from build123d import *
from build123d.topology import SkipClean

# Parameters (mm, degrees)
SKETCH2_W            = 55
SKETCH2_H            = 59
SKETCH2_R            = 1.6
SKETCH2_R_2          = 11
BOSS_EXTRUDE1_DEPTH  = 5
SKETCH4_W            = 5
SKETCH4_H            = 59
BOSS_EXTRUDE2_DEPTH  = 50
BOSS_EXTRUDE3_DEPTH  = 4
FILLET2_R            = 5
SKETCH7_W            = 5
SKETCH7_H            = 50
BOSS_EXTRUDE4_DEPTH  = 5
BOSS_EXTRUDE5_START  = -60
SKETCH8_W            = 5
SKETCH8_H            = 5
BOSS_EXTRUDE5_DEPTH  = 55
SKETCH10_R           = 2.25
SKETCH10_R_2         = 4.75
BOSS_EXTRUDE6_DEPTH  = 10
REVOLVE1_ANGLE       = 30
CIRPATTERN1_COUNT    = 2
CIRPATTERN1_ANGLE    = 270
MIRROR1_COPY_1_ANGLE = 30
CIRPATTERN2_COUNT    = 2
CIRPATTERN2_ANGLE    = 270
SKETCH12_R           = 14
SKETCH12_R_2         = 11
BOSS_EXTRUDE7_DEPTH  = 2
FILLET3_R            = 4
SKETCH14_W           = 5
SKETCH14_H           = 30
BOSS_EXTRUDE8_DEPTH  = 20
FILLET4_R            = 5
BOSS_EXTRUDE9_START  = 5
SKETCH15_W           = 51
SKETCH15_H           = 51
SKETCH15_R           = 1.6
SKETCH15_R_2         = 11
BOSS_EXTRUDE9_DEPTH  = 5


with BuildPart() as part:
    # Sketch2 → Boss-Extrude1 (new body)
    with BuildSketch(Plane.XY):
        with Locations((22.5, 22.5)):
            Rectangle(SKETCH2_W, SKETCH2_H)
        with Locations((0, 45)):
            Circle(SKETCH2_R, mode=Mode.SUBTRACT)
        with Locations((45, 45)):
            Circle(SKETCH2_R, mode=Mode.SUBTRACT)
        with Locations((45, 0)):
            Circle(SKETCH2_R, mode=Mode.SUBTRACT)
        Circle(SKETCH2_R, mode=Mode.SUBTRACT)
        with Locations((22.5, 22.5)):
            Circle(SKETCH2_R_2, mode=Mode.SUBTRACT)
    extrude(amount=BOSS_EXTRUDE1_DEPTH)

    # Sketch4 → Boss-Extrude2 (add)
    with BuildSketch(Plane(origin=(0, 0, 0), x_dir=(-1, 0, 0), z_dir=(0, 0, -1))):
        with Locations((7.5, 22.5)):
            Rectangle(SKETCH4_W, SKETCH4_H)
    extrude(amount=-BOSS_EXTRUDE2_DEPTH)

    # Sketch5 → Boss-Extrude3 (add)
    with BuildSketch(Plane(origin=(0, 52, 0), x_dir=(1, 0, 0), z_dir=(0, 1, 0))):
        Polygon((-5, -5), (8.512790644, -5), (-5, -18.512790644), align=None)
    boss_extrude3 = extrude(amount=-BOSS_EXTRUDE3_DEPTH)

    # Fillet2
    fillet2_edges = [part.edges().sort_by_distance(p)[0] for p in [
        (50, -7, 2.5),
    ]]
    fillet(fillet2_edges, radius=FILLET2_R)

    # Sketch7 → Boss-Extrude4 (add)
    with BuildSketch(Plane(origin=(0, 52, 0), x_dir=(1, 0, 0), z_dir=(0, 1, 0))):
        with Locations((-7.5, -25)):
            Rectangle(SKETCH7_W, SKETCH7_H)
    extrude(amount=BOSS_EXTRUDE4_DEPTH)

    # Sketch8 → Boss-Extrude5 (add)
    with BuildSketch(Plane.ZY.offset(10).offset(BOSS_EXTRUDE5_START)):
        with Locations((2.5, 54.5)):
            Rectangle(SKETCH8_W, SKETCH8_H)
    extrude(amount=BOSS_EXTRUDE5_DEPTH)

    # Sketch10 → Boss-Extrude6 (add)
    # profile 1 of 4: a face of its own
    with BuildSketch(Plane.XY.offset(5)):
        with BuildLine():
            Line((3.682729966, 48), (-3.682729966, 48))
            ThreePointArc((-3.682729966, 48), (0, 40.25), (3.682729966, 48))
        make_face()
        with Locations((0, 45)):
            Circle(SKETCH10_R, mode=Mode.SUBTRACT)
    # profile 2 of 4: a face of its own
    with BuildSketch(Plane.XY.offset(5)):
        with Locations((45, 45)):
            Circle(SKETCH10_R_2)
        with Locations((45, 45)):
            Circle(SKETCH10_R, mode=Mode.SUBTRACT)
    # profile 3 of 4: a face of its own
    with BuildSketch(Plane.XY.offset(5)):
        with Locations((45, 0)):
            Circle(SKETCH10_R_2)
        with Locations((45, 0)):
            Circle(SKETCH10_R, mode=Mode.SUBTRACT)
    # profile 4 of 4: a face of its own
    with BuildSketch(Plane.XY.offset(5)):
        Circle(SKETCH10_R_2)
        Circle(SKETCH10_R, mode=Mode.SUBTRACT)
    extrude(amount=BOSS_EXTRUDE6_DEPTH)

    # Sketch11 → Revolve1 (revolve, symmetric)
    with BuildSketch(Plane(origin=(0, 45, 0), x_dir=(0, 0, -1), z_dir=(0, 1, 0))) as revolve1_sk:
        Polygon((-5, -40.25), (-5, -35.032167456), (-11.67737913, -40.25), align=None)
    revolve1 = revolve(axis=Axis((45, 45, 15), (0, 0, -1)), revolution_arc=REVOLVE1_ANGLE / 2)
    revolve1 = revolve1 + revolve(revolve1_sk.sketch, axis=Axis((45, 45, 15), (0, 0, 1)), revolution_arc=REVOLVE1_ANGLE / 2)

    # CirPattern1: Revolve1 ×2 about axis
    cirpattern1_axis = Axis((45, 45, 15), (0, 0, -1))
    for i in range(1, CIRPATTERN1_COUNT):
        add(revolve1.rotate(cirpattern1_axis, i * CIRPATTERN1_ANGLE / (CIRPATTERN1_COUNT - 1)))

    # Mirror1: Revolve1 across plane
    add(revolve1.mirror(Plane.ZX.offset(22.5)))

    # Mirror1 copy 1 sketch → Mirror1 copy 1 (revolve, symmetric)
    with BuildSketch(Plane(origin=(45, 45, 0), x_dir=(0, 0, -1), z_dir=(-1, 0, 0))) as mirror1_copy_1_sk:
        Polygon((-5, 40.25), (-5, 35.032167456), (-11.67737913, 40.25), align=None)
    revolve(axis=Axis((45, 0, 15), (0, 0, 1)), revolution_arc=MIRROR1_COPY_1_ANGLE / 2)
    revolve(mirror1_copy_1_sk.sketch, axis=Axis((45, 0, 15), (0, 0, -1)), revolution_arc=MIRROR1_COPY_1_ANGLE / 2)

    # CirPattern2: Revolve1 ×2 about axis
    cirpattern2_axis = Axis((45, 45, 15), (0, 0, 1))
    for i in range(1, CIRPATTERN2_COUNT):
        add(revolve1.rotate(cirpattern2_axis, i * CIRPATTERN2_ANGLE / (CIRPATTERN2_COUNT - 1)))

    # Sketch12 → Boss-Extrude7 (add)
    with BuildSketch(Plane.XY.offset(5)):
        with Locations((22.5, 22.5)):
            Circle(SKETCH12_R)
        with Locations((22.5, 22.5)):
            Circle(SKETCH12_R_2, mode=Mode.SUBTRACT)
    extrude(amount=BOSS_EXTRUDE7_DEPTH)

    # Mirror2: Boss-Extrude3 across plane
    add(boss_extrude3.mirror(Plane.ZX.offset(22.5)))

    # Fillet3
    fillet3_edges = [part.edges().sort_by_distance(p)[0] for p in [
        (40.411852325, 43.770609536, 8.338689565),
        (40.411852325, 46.229390464, 8.338689565),
        (46.229390464, 40.411852325, 8.338689565),
        (43.770609536, 40.411852325, 8.338689565),
        (40.411852325, -1.229390464, 8.338689565),
        (40.411852325, 1.229390464, 8.338689565),
        (43.770609536, 4.588147675, 8.338689565),
        (46.229390464, 4.588147675, 8.338689565),
        (43.770609536, 49.588147675, 8.338689565),
        (46.229390464, 49.588147675, 8.338689565),
    ]]
    fillet(fillet3_edges, radius=FILLET3_R)

    # Sketch14 → Boss-Extrude8 (add)
    with BuildSketch(Plane(origin=(0, 57, 0), x_dir=(1, 0, 0), z_dir=(0, 1, 0))):
        with Locations((-7.5, -35)):
            Rectangle(SKETCH14_W, SKETCH14_H)
    extrude(amount=BOSS_EXTRUDE8_DEPTH)

    # Fillet4
    fillet4_edges = [part.edges().sort_by_distance(p)[0] for p in [
        (-5, 22.5, 5),
    ]]
    fillet(fillet4_edges, radius=FILLET4_R)

    # Sketch15 → Boss-Extrude9 (add)
    with SkipClean():  # the faces are left unmerged after this step: merging them gives an invalid solid
        with BuildSketch(Plane(origin=(0, 0, 0), x_dir=(-1, 0, 0), z_dir=(0, 0, -1)).offset(BOSS_EXTRUDE9_START)):
            with Locations((-22.5, 22.5)):
                Rectangle(SKETCH15_W, SKETCH15_H)
            Circle(SKETCH15_R, mode=Mode.SUBTRACT)
            with Locations((0, 45)):
                Circle(SKETCH15_R, mode=Mode.SUBTRACT)
            with Locations((-45, 45)):
                Circle(SKETCH15_R, mode=Mode.SUBTRACT)
            with Locations((-45, 0)):
                Circle(SKETCH15_R, mode=Mode.SUBTRACT)
            with Locations((-22.5, 22.5)):
                Circle(SKETCH15_R_2, mode=Mode.SUBTRACT)
        extrude(amount=-BOSS_EXTRUDE9_DEPTH)


solid = part.part
Check sheet for the modelled part. Datum: model origin and axes. Units: mm. A direction names the side the tool comes from. Coordinates: 2 decimals unless noted, no trailing zeros. Loops run counter-clockwise (first coordinate to the right, second up) from the corner with the lowest first, then second, coordinate; pieces in that order, holes last. Notation, with made-up numbers: (-7.5, -2) -> (1.5, -2) arc R31 ccw to (1.5, 30) -> close; hole circle Ø2 at (71, 22). An arc over 180 degrees is marked (long way). Answer in a Markdown table with one row per item.
1. Sectioned sample at A-A, the plane x = 22.5. Record the boundary of the cut face in (y, z), then the cut area to 3 significant figures.
Check values:
| item | result |
|---|---|
| outline | (-7, 0) -> (-3, 0) -> (-3, -5) -> (11.5, -5) -> (11.5, 7) -> (8.5, 7) -> (8.5, 5) -> (-7, 5) -> close; (33.5, -5) -> (48, -5) -> (48, 0) -> (57, 0) -> (57, 5) -> (36.5, 5) -> (36.5, 7) -> (33.5, 7) -> close |
| area | 367 mm2 |
2. Material ranges on line 1 along Y through (x, z) = (45, 2); line 2 along X through (y, z) = (0, 1.9); line 3 along Y through (x, z) = (0, -3), recorded low to high. Write a range as [from, to].
Check values:
| item | result |
|---|---|
| line 1 | y = [-7, -1.6], [1.6, 43.4], [46.6, 57] |
| line 2 | x = [-10, -1.6], [1.6, 43.4], [46.6, 50] |
| line 3 | y = [-3, -1.6], [1.6, 43.4], [46.6, 48] |
3. Go/stop test with flat-tipped pins: pin 1 (5 mm diameter, centred on x = 1.5, y = 2, fed in from +Z); pin 2 (16 mm diameter, centred on x = 10, z = 14, fed in from +Y); pin 3 (2.5 mm diameter, centred on x = 0, y = 45, fed in from -Z); pin 4 (4 mm diameter, centred on y = 2, z = 27.5, fed in from +X). Record where each tip stops, or that it passes through.
Check values:
| item | result |
|---|---|
| pin 1 | stops at z = 15 |
| pin 2 | stops at y = 52 |
| pin 3 | passes through |
| pin 4 | stops at x = -5 |
4. Sectioned sample at B-B, the plane y = 22.5. Record the boundary of the cut face in (x, z), then the cut area to 3 significant figures.
Check values:
| item | result |
|---|---|
| outline | (-10, 0) -> (-3, 0) -> (-3, -5) -> (11.5, -5) -> (11.5, 7) -> (8.5, 7) -> (8.5, 5) -> (0, 5) arc R5 cw to (-5, 10) -> (-5, 50) -> (-10, 50) -> close; (33.5, -5) -> (48, -5) -> (48, 0) -> (50, 0) -> (50, 5) -> (36.5, 5) -> (36.5, 7) -> (33.5, 7) -> close |
| area | 577 mm2 |
5. Sectioned sample at C-C, the plane z = 44.5. Record the boundary of the cut face in (x, y).
Check values:
| item | result |
|---|---|
| outline | (-10, -7) -> (-5, -7) -> (-5, 77) -> (-10, 77) -> close |
6. Access from +Z, -Z, +X, -X, +Y, -Y to the whole of each face (thin tool, end or side, straight path). Record for faces 1 (the face through (0, 42, 15)), 2 (the face through (-10, 34, 25)), 3 (the face through (49.388, -1.819, 11.041)), 4 (the face through (2, 48, 14)).
Check values:
| item | result |
|---|---|
| face 1 | +Z, +X |
| face 2 | +Z, -Z, -X, +Y, -Y |
| face 3 | +Z |
| face 4 | +Z, +Y |
